The model under review builds one solid part; all positions refer to its coordinate system, in mm. Face numbers are marked on the shaded views. A direction names the side the tool comes from. Round coordinates to 2 decimals unless told otherwise and drop trailing zeros. Write each loop counter-clockwise with the first axis right and the second up, starting at its lowest first coordinate (ties: lowest second). Pieces come first, ordered by that corner, then holes. Notation, with made-up numbers: (76, -10) -> (119, -10) arc R23 ccw to (119, 12) -> close; hole circle Ø11 at (59.5, 33). An arc over 180 degrees is marked (long way). Answer as a JSON object with one key per item and string values. Group by question number.
1) To check wall thickness, follow probe 1 along Y at (x, z) = (27, 28.5) (3 decimals). State the ranges of the line that lie inside material, in increasing order. Write a range as [from, to].
2) We need section C-C, the plane z = -19.5. Write out the cut boundary in (x, y) (3 decimals).
3) We need section A-A, the plane x = -33. Write out the cut boundary in (y, z) (3 decimals).
4) Machinability: for the marked faces 4 and 5, which of the approach directions +Z, -Z, +X, -X, +Y, -Y give a long, thin tool a straight path to every point of the face, cutting with its end or side? Answer none if there is none.
5) Mouldability with a two-part tool opening along X and no side actions: class the marked faces 1, 2 and 3 as pulls with the +X half, pulls with the -X half, needs draft (parallel to the pull), parting line crosses it, or undercut.
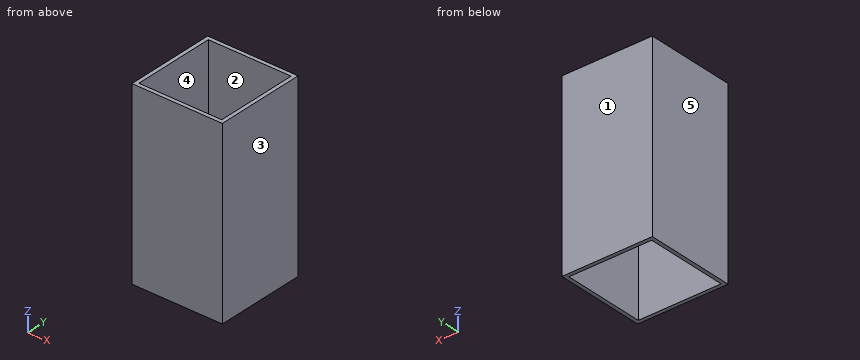
from build123d import *

# Parameters (mm, degrees)
SKETCH3_W                = 76.2
SKETCH3_H                = 76.2
SKETCH3_W_2              = 69.85
SKETCH3_H_2              = 69.85
BOSS_EXTRUDE1_DEPTH      = 76.2
BOSS_EXTRUDE1_DEPTH_BACK = 76.2


with BuildPart() as part:
    # Sketch3 → Boss-Extrude1 (new body, two sides)
    with BuildSketch(Plane.XY) as boss_extrude1_sk:
        Rectangle(SKETCH3_W, SKETCH3_H)
        Rectangle(SKETCH3_W_2, SKETCH3_H_2, mode=Mode.SUBTRACT)
    extrude(amount=BOSS_EXTRUDE1_DEPTH)
    extrude(boss_extrude1_sk.sketch, amount=-BOSS_EXTRUDE1_DEPTH_BACK)


solid = part.part
Here are the results:
{
 "1": {"probe 1": "y = [-38.1, -34.925], [34.925, 38.1]"},
 "2": {"outline": "(-38.1, -38.1) -> (38.1, -38.1) -> (38.1, 38.1) -> (-38.1, 38.1) -> close; hole (-34.925, -34.925) -> (34.925, -34.925) -> (34.925, 34.925) -> (-34.925, 34.925) -> close"},
 "3": {"outline": "(-38.1, -76.2) -> (-34.925, -76.2) -> (-34.925, 76.2) -> (-38.1, 76.2) -> close; (34.925, -76.2) -> (38.1, -76.2) -> (38.1, 76.2) -> (34.925, 76.2) -> close"},
 "4": {"face 4": "+Z, -Z", "face 5": "+Z, -Z, -X, +Y, -Y"},
 "5": {"face 1": "needs draft", "face 2": "undercut", "face 3": "pulls with the +X half"}
}
